Part model, mm, in its own coordinate system. Face numbers are marked on the shaded views. A direction names the side the tool comes from. Round coordinates to 2 decimals unless told otherwise and drop trailing zeros. Write each loop counter-clockwise with the first axis right and the second up, starting at its lowest first coordinate (ties: lowest second). Pieces come first, ordered by that corner, then holes. Notation, with made-up numbers: (-27, 10) -> (-13, 10) arc R27 ccw to (-13, 43) -> close; hole circle Ø9 at (87, 3.25). An arc over 180 degrees is marked (long way). Return JSON: item names as keys, results as strings. Group by question number.
(1) Saw through at A-A (x = 0). List the corners of the cut face in (y, z), plus the area to 4 significant figures.
(2) Tool access for the marked faces 1 and 2: list every direction of +Z, -Z, +X, -X, +Y, -Y with a clear straight run to the whole face (end or side of a thin tool).
(3) Saw through at D-D (x = -14.5). List the corners of the cut face in (y, z), plus the area to 4 significant figures.
(4) Saw through at C-C (z = 36). List the corners of the cut face in (x, y), plus the area to 3 significant figures.
(5) Drop flat-ended pins along their axis: pin 1 Ø8 at (x, y) = (-8.5, 11.5) entering from +Z; pin 2 Ø10 at (y, z) = (0, 40) entering from -X. Give the stop position or say it passes through.
(6) Drill centre lines: L1, parallel to Z at x = 4.5, y = -8; L2, parallel to Y at x = 0, z = 41; L3, parallel to X at y = 1.5, z = 48.5. Where is each one in solid material? Low to high. Write a range as from..to.
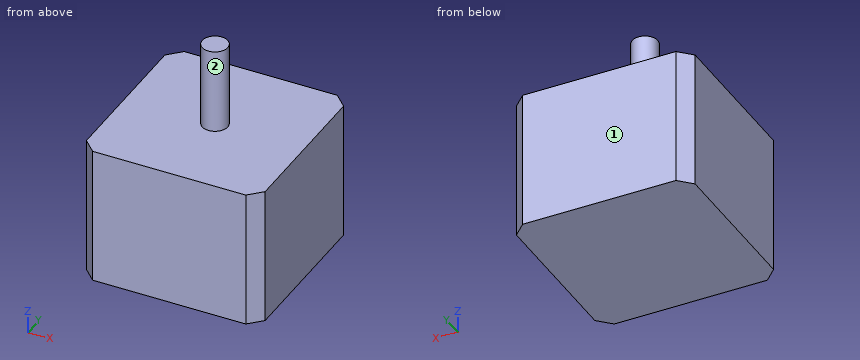
from build123d import *

# Parameters (mm, degrees)
SKETCH1_W           = 42
SKETCH1_H           = 42
BOSS_EXTRUDE1_DEPTH = 32.5
CHAMFER1_SIZE       = 3
SKETCH2_R           = 3
BOSS_EXTRUDE2_DEPTH = 20


with BuildPart() as part:
    # Sketch1 → Boss-Extrude1 (new body)
    with BuildSketch(Plane(origin=(0, 0, 0), x_dir=(0, 1, 0), z_dir=(0, 0, 1))):
        Rectangle(SKETCH1_W, SKETCH1_H)
    extrude(amount=BOSS_EXTRUDE1_DEPTH)

    # Chamfer1
    chamfer1_edges = [part.edges().sort_by_distance(p)[0] for p in [
        (21, 21, 16.25),
        (21, -21, 16.25),
        (-21, -21, 16.25),
        (-21, 21, 16.25),
    ]]
    chamfer(chamfer1_edges, length=CHAMFER1_SIZE)

    # Sketch2 → Boss-Extrude2 (add)
    with BuildSketch(Plane.XY.offset(32.5)):
        Circle(SKETCH2_R)
    extrude(amount=BOSS_EXTRUDE2_DEPTH)


solid = part.part
Computed values:
{
 "1": {"outline": "(-21, 0) -> (21, 0) -> (21, 32.5) -> (3, 32.5) -> (3, 52.5) -> (-3, 52.5) -> (-3, 32.5) -> (-21, 32.5) -> close", "area": "1,485 mm2"},
 "2": {"face 1": "+Z, -Z, +X, -X, +Y", "face 2": "+Z"},
 "3": {"outline": "(-21, 0) -> (21, 0) -> (21, 32.5) -> (-21, 32.5) -> close", "area": "1,365 mm2"},
 "4": {"outline": "circle Ø6 at (0, 0)", "area": "28.3 mm2"},
 "5": {"pin 1": "z = 32.5", "pin 2": "x = -3"},
 "6": {"L1": "0..32.5", "L2": "-3..3", "L3": "-2.6..2.6"}
}
